Geometry check sheet. Reference: drawing and pictorial views, mm from the part's lowest x, y, z. A direction names the side the tool comes from. Round coordinates to 2 decimals unless told otherwise and drop trailing zeros. Order: outer loops, then holes, each group sorted by start corner. A loop starts at its lowest first (then second) coordinate and runs counter-clockwise, first axis right, second up. Notation, with made-up numbers: (-12, 13) -> (47, 13) arc R31 cw to (47, 43) -> close; hole circle Ø2 at (32.25, -36.75). An arc over 180 degrees is marked (long way). Return JSON: item names as keys, results as strings. Group by question number.
1) Section check D-D on z = 5. Enter the section's corners in (x, y).
2) Tool access check on the marked faces 1 and 2. Record the directions out of +Z, -Z, +X, -X, +Y, -Y that give a thin tool (end or side, any length) a straight path to the whole face; none if there is none.
3) Section check B-B on z = 6.5. Enter the section's corners in (x, y).
4) Depth check by flat-ended pin: pin 1 (1.5 mm diameter, centred on y = 20.5, z = 4, fed in from +X); pin 2 (1.5 mm diameter, centred on x = 13.5, z = 7.5, fed in from +Y). Enter the tip coordinate at first touch or a pass-through.
5) Section check A-A on y = 17. Enter the section's corners in (x, z), plus the area to 3 significant figures.
6) Scan lines: L1, parallel to Z at x = 0.4, y = 17; L2, parallel to X at y = 1.3, z = 6.5; L3, parallel to X at y = 20, z = 6.5. Record each from-to range of solid material in increasing order.
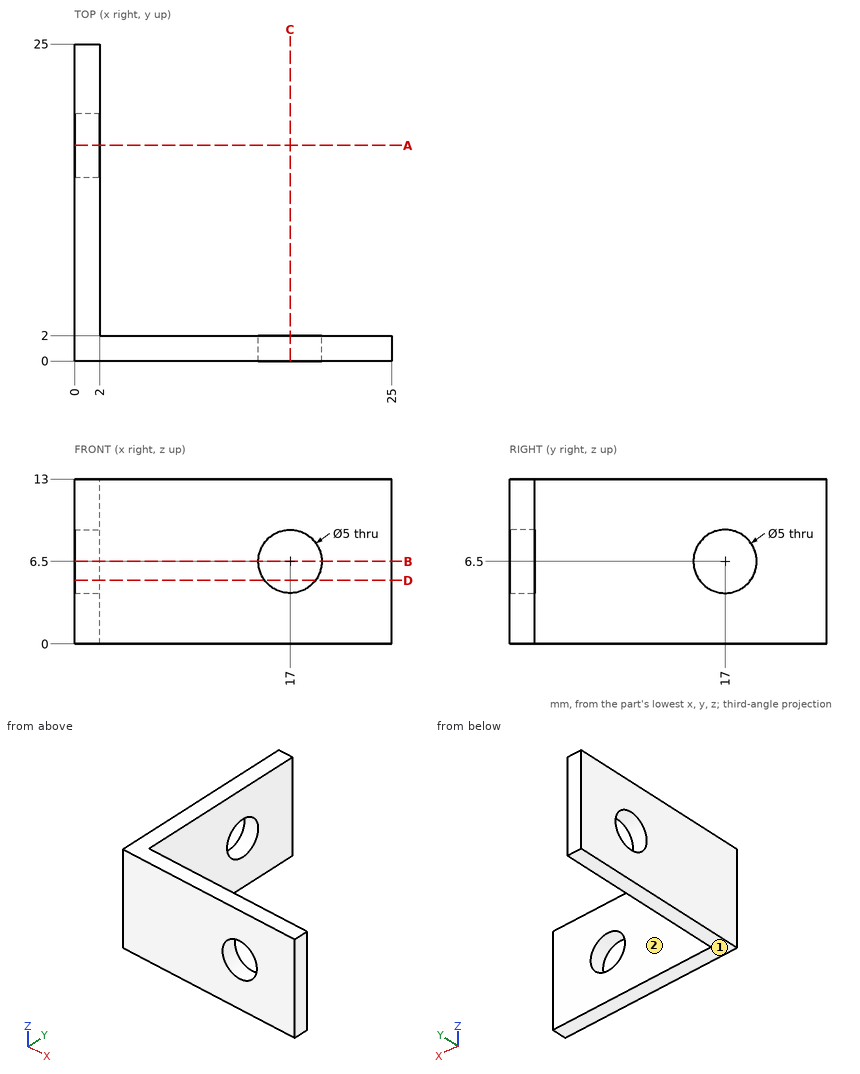
Check result:
{
 "1": {"outline": "(0, 0) -> (15, 0) -> (15, 2) -> (2, 2) -> (2, 15) -> (0, 15) -> close; (0, 19) -> (2, 19) -> (2, 25) -> (0, 25) -> close; (19, 0) -> (25, 0) -> (25, 2) -> (19, 2) -> close"},
 "2": {"face 1": "-Z, +X, -X, +Y, -Y", "face 2": "+Z, -Z, +X, +Y"},
 "3": {"outline": "(0, 0) -> (14.5, 0) -> (14.5, 2) -> (2, 2) -> (2, 14.5) -> (0, 14.5) -> close; (0, 19.5) -> (2, 19.5) -> (2, 25) -> (0, 25) -> close; (19.5, 0) -> (25, 0) -> (25, 2) -> (19.5, 2) -> close"},
 "4": {"pin 1": "x = 2", "pin 2": "y = 2"},
 "5": {"outline": "(0, 0) -> (2, 0) -> (2, 4) -> (0, 4) -> close; (0, 9) -> (2, 9) -> (2, 13) -> (0, 13) -> close", "area": "16.0 mm^2"},
 "6": {"L1": "0 to 4, 9 to 13", "L2": "0 to 14.5, 19.5 to 25", "L3": "0 to 2"}
}
